```python
from build123d import *

# Parameters (mm, degrees)
BASE_FLANGE1_DEPTH           = 3.175
EDGE_FLANGE1_START           = -833.4375
EDGE_FLANGE1_DEPTH           = 600.075
EDGE_FLANGE1_2_DEPTH         = 1.5875
EDGE_FLANGE1_START_2         = -234.95
EDGE_FLANGE1_3_DEPTH         = 1.5875
EDGE_FLANGE1_START_3         = -831.85
EDGE_FLANGE1_4_DEPTH         = 596.9
SKETCH10_R                   = 4.3688
CUT_EXTRUDE1_DEPTH           = 1070.608165207
SKETCH11_R                   = 2.45745
CUT_EXTRUDE2_DEPTH           = 1071.515830826
EDGE_FLANGE2_STRIP_W         = 19.05
EDGE_FLANGE2_STRIP_H         = 3.175
EDGE_FLANGE2_STRIP_CUT_DEPTH = 1066.8
EDGE_FLANGE2_DEPTH           = 1066.8
FILLET1_R                    = 6.35


# Read off the part's stored shape, not the designer's step: Edge-Flange1
# Sheet-metal steps are written as plain solids
with BuildPart() as part:
    # Sketch1 → Base-Flange1 (new body)
    with BuildSketch(Plane(origin=(0, 0, 0), x_dir=(0, 0, -1), z_dir=(1, 0, 0))):
        Polygon((838.2, 0), (1066.8, 0), (1066.8, 73.025), (0, 73.025), (0, 0), (228.6, 0), (228.6, 12.7), (234.95, 12.7), (234.95, 11.43), (831.85, 11.43), (831.85, 12.7), (838.2, 12.7), align=None)
    extrude(amount=-BASE_FLANGE1_DEPTH)

    # Edge-Flange1 outline → Edge-Flange1 (cut)
    with BuildSketch(Plane.XY.offset(EDGE_FLANGE1_START)):
        with BuildLine():
            Line((-3.175, 16.929261314), (-3.175, 11.43))
            Line((-3.175, 11.43), (0, 11.43))
            ThreePointArc((0, 11.43), (-2.324261314, 13.754261314), (-3.175, 16.929261314))
        make_face()
    extrude(amount=EDGE_FLANGE1_DEPTH, mode=Mode.SUBTRACT)

    # Edge-Flange1 2 outline → Edge-Flange1 2 (cut)
    with BuildSketch(Plane.XY.offset(EDGE_FLANGE1_START)):
        with BuildLine():
            Line((0, 18.516761314), (-3.175, 18.516761314))
            Line((-3.175, 18.516761314), (-3.175, 16.929261314))
            ThreePointArc((-3.175, 16.929261314), (-2.757968249, 14.665992052), (-1.561649527, 12.7))
            Line((-1.561649527, 12.7), (0, 12.7))
            Line((0, 12.7), (0, 18.516761314))
        make_face()
    extrude(amount=EDGE_FLANGE1_2_DEPTH, mode=Mode.SUBTRACT)

    # Edge-Flange1 3 outline → Edge-Flange1 3 (cut)
    with BuildSketch(Plane.XY.offset(EDGE_FLANGE1_START_2)):
        with BuildLine():
            Line((0, 18.516761314), (-3.175, 18.516761314))
            Line((-3.175, 18.516761314), (-3.175, 16.929261314))
            ThreePointArc((-3.175, 16.929261314), (-2.757968249, 14.665992052), (-1.561649527, 12.7))
            Line((-1.561649527, 12.7), (0, 12.7))
            Line((0, 12.7), (0, 18.516761314))
        make_face()
    extrude(amount=EDGE_FLANGE1_3_DEPTH, mode=Mode.SUBTRACT)

    # Edge-Flange1 4 outline → Edge-Flange1 4 (add)
    with BuildSketch(Plane.XY.offset(EDGE_FLANGE1_START_3)):
        with BuildLine():
            ThreePointArc((1.5875, 14.179630657), (0.425369343, 15.341761314), (0, 16.929261314))
            Line((0, 16.929261314), (0, 11.43))
            Line((0, 11.43), (46.318351826, -15.311912895))
            Line((46.318351826, -15.311912895), (47.905851826, -12.562282238))
            Line((47.905851826, -12.562282238), (1.5875, 14.179630657))
        make_face()
    extrude(amount=EDGE_FLANGE1_4_DEPTH)

    # Sketch10 → Cut-Extrude1 (cut, through all)
    with BuildSketch(Plane(origin=(4.949335183, 8.5725, 0), x_dir=(0.8660254037844364, -0.5000000000000041, 0), z_dir=(-0.500000000000004, -0.8660254037844363, 0))):
        with Locations((22.112285791, -285.75)):
            Circle(SKETCH10_R)
        with Locations((22.112285791, -781.05)):
            Circle(SKETCH10_R)
    extrude(amount=-CUT_EXTRUDE1_DEPTH, mode=Mode.SUBTRACT)

    # Sketch11 → Cut-Extrude2 (cut, through all)
    with BuildSketch(Plane.ZY.offset(3.175)):
        with Locations((-1038.225, 60.325)):
            Circle(SKETCH11_R)
        with Locations((-866.775, 60.325)):
            Circle(SKETCH11_R)
        with Locations((-1038.225, 12.7)):
            Circle(SKETCH11_R)
        with Locations((-866.775, 12.7)):
            Circle(SKETCH11_R)
        with Locations((-200.025, 60.325)):
            Circle(SKETCH11_R)
        with Locations((-200.025, 12.7)):
            Circle(SKETCH11_R)
        with Locations((-28.575, 12.7)):
            Circle(SKETCH11_R)
        with Locations((-28.575, 60.325)):
            Circle(SKETCH11_R)
    extrude(amount=-CUT_EXTRUDE2_DEPTH, mode=Mode.SUBTRACT)

    # Edge-Flange2 strip (across the edge) → Edge-Flange2 strip cut (cut)
    with BuildSketch(Plane(origin=(0, 73.025, -1066.8), x_dir=(0, -1, 0), z_dir=(0, 0, 1))):
        with Locations((-3.175, -1.5875)):
            Rectangle(EDGE_FLANGE2_STRIP_W, EDGE_FLANGE2_STRIP_H)
    extrude(amount=EDGE_FLANGE2_STRIP_CUT_DEPTH, mode=Mode.SUBTRACT)

    # Edge-Flange2 section (across the edge) → Edge-Flange2 (add)
    with BuildSketch(Plane(origin=(0, 73.025, -1066.8), x_dir=(0, -1, 0), z_dir=(0, 0, 1))):
        with BuildLine():
            Line((0, 3.175), (0, 9.525))
            Line((0, 9.525), (3.175, 9.525))
            Line((3.175, 9.525), (3.175, 3.175))
            ThreePointArc((3.175, 3.175), (4.10493597, 0.92993597), (6.35, 0))
            Line((6.35, 0), (6.35, -3.175))
            ThreePointArc((6.35, -3.175), (1.859871939, -1.315128061), (0, 3.175))
        make_face()
    extrude(amount=EDGE_FLANGE2_DEPTH)

    # Fillet1
    fillet1_edges = [part.edges().sort_by_distance(p)[0] for p in [
        (-1.5875, 0, 0),
        (47.112101826, -13.937097567, -234.95),
        (-1.5875, 0, -228.6),
        (47.112101826, -13.937097567, -831.85),
        (-1.5875, 0, -838.2),
        (-1.5875, 0, -1066.8),
        (9.525, 71.4375, 0),
        (9.525, 71.4375, -1066.8),
    ]]
    fillet(fillet1_edges, radius=FILLET1_R)


solid = part.part
```
The listing builds one solid part. Answer for the finished solid, in the listing's coordinates (mm). Coordinates: 2 decimals unless noted, no trailing zeros. Write each loop counter-clockwise with the first axis right and the second up, starting at its lowest first coordinate (ties: lowest second). Pieces come first, ordered by that corner, then holes.
Q1. Section A-A, the plane z = -160.5 is taken. Write down the section's boundary in (x, y) (3 decimals), then the cut area to 3 significant figures.
Returned:
outline: (-3.175, 0) - (0, 0) - (0, 66.675) arc R3.175 cw to (3.175, 69.85) - (9.525, 69.85) - (9.525, 73.025) - (3.175, 73.025) arc R6.35 ccw to (-3.175, 66.675) - close
area: 256 mm2
Q2. The mould has two halves that part along Y. Classify faces 1 (the flat face through (18, 2, -234.95)), 2 (the flat face through (0, 34, -526)), 3 (the flat face through (22.83, -1.75, -537.58)): released by +Y, released by -Y, zero draft, split by the parting line, or undercut.
Returned:
face 1: zero draft
face 2: undercut
face 3: released by -Y
Q3. Given P1, Ø1.5, axis at y = 26, z = -716, coming from the +X side; P2, Ø2.5, axis at x = -2, z = -931, coming from the -Y side; P3, Ø3.5, axis at x = -2, z = -835.5, coming from the -Y side, each flat-ended and moving along its own axis, determine where each tip first touches the part or whether it passes through.
Returned:
P1: stops at x = 0
P2: stops at y = 0
P3: stops at y = 12.7
Q4. Find the intervals of material crossed by line 1 along Z through (x, y) = (-1, 12); line 2 along X through (y, z) = (22, -248) (3 decimals); line 3 along Z through (x, y) = (29, -5), in increasing order.
Returned:
line 1: z = -1066.8 to -1040.58, -1035.87 to -869.13, -864.42 to -838.2, -228.6 to -202.38, -197.67 to -30.93, -26.22 to 0
line 2: x = -3.175 to 0
line 3: z = -831.85 to -234.95
